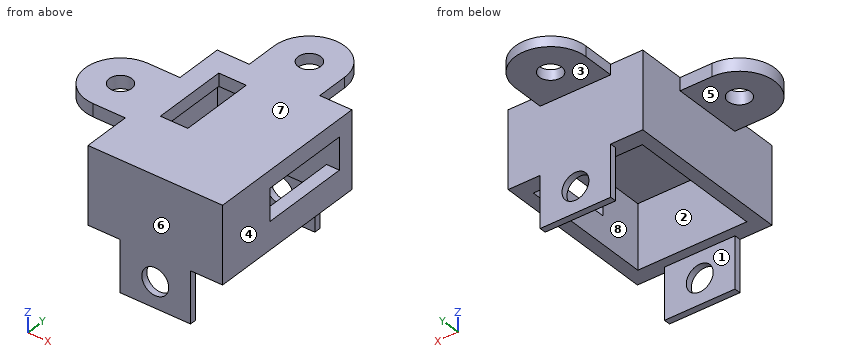
from build123d import *

# Parameters (mm, degrees)
SKETCH1_W           = 21
SKETCH1_H           = 26
SKETCH1_W_2         = 17
SKETCH1_H_2         = 21
BOSS_EXTRUDE1_DEPTH = 10
SKETCH2_W           = 21
SKETCH2_H           = 26
BOSS_EXTRUDE2_DEPTH = 2
SKETCH4_W           = 5
SKETCH4_H           = 14
CUT_EXTRUDE2_DEPTH  = 2
SKETCH6_R           = 1.76
BOSS_EXTRUDE3_DEPTH = 1.6
SKETCH9_R           = 1.76
BOSS_EXTRUDE5_DEPTH = 2
SKETCH14_W          = 11
SKETCH14_H          = 1
BOSS_EXTRUDE8_DEPTH = 8
SKETCH16_R          = 2.1
CUT_EXTRUDE3_DEPTH  = 39
CUT_EXTRUDE4_DEPTH  = 10
SKETCH18_R          = 1.75
BOSS_EXTRUDE9_DEPTH = 2
SKETCH19_W          = 4.280254221
SKETCH19_H          = 11.747931796
CUT_EXTRUDE5_DEPTH  = 10


with BuildPart() as part:
    # Sketch1 → Boss-Extrude1 (new body)
    with BuildSketch(Plane.XY):
        Rectangle(SKETCH1_W, SKETCH1_H)
        Rectangle(SKETCH1_W_2, SKETCH1_H_2, mode=Mode.SUBTRACT)
    extrude(amount=BOSS_EXTRUDE1_DEPTH)

    # Sketch2 → Boss-Extrude2 (add)
    with BuildSketch(Plane.XY.offset(10)):
        Rectangle(SKETCH2_W, SKETCH2_H)
    extrude(amount=BOSS_EXTRUDE2_DEPTH)

    # Sketch4 → Cut-Extrude2 (cut)
    with BuildSketch(Plane(origin=(10.5, 0, 0), x_dir=(0, 0, -1), z_dir=(1, 0, 0))):
        with Locations((-6.8, 3.5)):
            Rectangle(SKETCH4_W, SKETCH4_H)
    extrude(amount=-CUT_EXTRUDE2_DEPTH, mode=Mode.SUBTRACT)

    # Sketch6 → Boss-Extrude3 (add)
    with BuildSketch(Plane.XY.offset(12)):
        with BuildLine():
            Line((0, 13), (5.5, 13))
            Line((5.5, 13), (5.5, 18))
            ThreePointArc((5.5, 18), (0, 23.5), (-5.5, 18))
            Line((-5.5, 18), (-5.5, 13))
            Line((-5.5, 13), (0, 13))
        make_face()
        with Locations((0, 18)):
            Circle(SKETCH6_R, mode=Mode.SUBTRACT)
    extrude(amount=-BOSS_EXTRUDE3_DEPTH)

    # Sketch9 → Boss-Extrude5 (add)
    with BuildSketch(Plane.XY.offset(12)):
        with BuildLine():
            Line((0, -13), (-5.5, -13))
            Line((-5.5, -13), (-5.5, -18))
            ThreePointArc((-5.5, -18), (0, -23.5), (5.5, -18))
            Line((5.5, -18), (5.5, -13))
            Line((5.5, -13), (0, -13))
        make_face()
        with Locations((0, -18)):
            Circle(SKETCH9_R, mode=Mode.SUBTRACT)
    extrude(amount=-BOSS_EXTRUDE5_DEPTH)

    # Sketch14 → Boss-Extrude8 (add)
    with BuildSketch(Plane(origin=(0, 0, 0), x_dir=(-1, 0, 0), z_dir=(0, 0, -1))):
        with Locations((0, -12.5)):
            Rectangle(SKETCH14_W, SKETCH14_H)
        with Locations((0, 12.5)):
            Rectangle(SKETCH14_W, SKETCH14_H)
    extrude(amount=BOSS_EXTRUDE8_DEPTH)

    # Sketch16 → Cut-Extrude3 (cut)
    with BuildSketch(Plane(origin=(0, 13, 0), x_dir=(1, 0, 0), z_dir=(0, 1, 0))):
        with Locations((0, 4)):
            Circle(SKETCH16_R)
    extrude(amount=-CUT_EXTRUDE3_DEPTH, mode=Mode.SUBTRACT)

    # Sketch17 → Cut-Extrude4 (cut)
    with BuildSketch(Plane(origin=(0, 0, 10), x_dir=(-1, 0, 0), z_dir=(0, 0, -1))):
        with BuildLine():
            Line((-5.5, -18), (-5.5, -13))
            Line((-5.5, -13), (5.5, -13))
            Line((5.5, -13), (5.5, -18))
            ThreePointArc((5.5, -18), (0, -23.5), (-5.5, -18))
        make_face()
    extrude(amount=-CUT_EXTRUDE4_DEPTH, mode=Mode.SUBTRACT)

    # Sketch18 → Boss-Extrude9 (add)
    with BuildSketch(Plane.XY.offset(12)):
        with BuildLine():
            Line((-10.5, 0), (-10.5, 5.5))
            Line((-10.5, 5.5), (-15.5, 5.5))
            ThreePointArc((-15.5, 5.5), (-21, 0), (-15.5, -5.5))
            Line((-15.5, -5.5), (-10.5, -5.5))
            Line((-10.5, -5.5), (-10.5, 0))
        make_face()
        with Locations((-15.5, 0)):
            Circle(SKETCH18_R, mode=Mode.SUBTRACT)
    extrude(amount=-BOSS_EXTRUDE9_DEPTH)

    # Sketch19 → Cut-Extrude5 (cut)
    with BuildSketch(Plane(origin=(0, 0, 10), x_dir=(-1, 0, 0), z_dir=(0, 0, -1))):
        with Locations((5.165781479, 3.32004636)):
            Rectangle(SKETCH19_W, SKETCH19_H)
    extrude(amount=-CUT_EXTRUDE5_DEPTH, mode=Mode.SUBTRACT)


solid = part.part
Read the model definition and answer for the solid it produces. Units are mm, in the model's axes. Face numbers are marked on the shaded views. A direction names the side the tool comes from. Round coordinates to 2 decimals unless told otherwise and drop trailing zeros. Loops run counter-clockwise (first coordinate to the right, second up) from the corner with the lowest first, then second, coordinate; pieces in that order, holes last. Notation, with made-up numbers: (-0.5, 46) - (5.5, 46) arc R14 ccw to (5.5, 64) - close; hole circle Ø10 at (39, -5). An arc over 180 degrees is marked (long way). One line per question, with ' | ' between items. Start each with the question number.
Q1. For the marked faces 1, 2, 3, 4 and 5, determine the directions among +Z, -Z, +X, -X, +Y, -Y from which every point of the face is accessible in a straight line to the end or side of a thin tool.
Q2. Section D-D on x = 8 is taken. Give the vertices of the cut face in (y, z), plus the area to 3 significant figures.
Q3. For a pull along Y with two mould halves and no side action, classify the marked faces 6, 7 and 8 as +Y half, -Y half, draft (parallel to the pull), parting line (faces both ways), or undercut.
Q4. Section C-C on y = 4 is taken. Give the vertices of the cut face in (x, z).
Q5. Find the intervals of material crossed by L1, parallel to Y at x = -1, z = 9.5; L2, parallel to Z at x = 0, y = -12.35; L3, parallel to Y at x = -15.5, z = 10.95, in increasing order.
Q6. Section B-B on z = -3.25 is taken. Give the vertices of the cut face in (x, y), plus the area to 3 significant figures.
Q7. Section A-A on y = 0 is taken. Give the vertices of the cut face in (x, z), plus the area to 3 significant figures.
Q8. Flat-ended cylindrical pins translate along their axes: pin 1 (9 mm diameter, centred on x = 1.5, z = -5.5, fed in from +Y); pin 2 (1.5 mm diameter, centred on x = -10.5, y = -3.5, fed in from -Z); pin 3 (1 mm diameter, centred on x = -13, z = 11, fed in from +Y). Find the tip coordinate at first contact, or state that the pin passes through.
Established:
1) face 1: -Z, +X, -X | face 2: -Z | face 3: -Z, +X, -X, +Y | face 4: +Z, -Z, +X, +Y, -Y | face 5: -Z, -X, +Y, -Y
2) outline: (-13, 0) - (-10.5, 0) - (-10.5, 10) - (10.5, 10) - (10.5, 0) - (13, 0) - (13, 12) - (-13, 12) - close | area: 102 mm²
3) face 6: -Y half | face 7: draft | face 8: undercut
4) outline: (-19.27, 10) - (-10.5, 10) - (-10.5, 0) - (-8.5, 0) - (-8.5, 10) - (-7.31, 10) - (-7.31, 12) - (-19.27, 12) - close; (-3.03, 10) - (8.5, 10) - (8.5, 9.3) - (10.5, 9.3) - (10.5, 12) - (-3.03, 12) - close; (8.5, 0) - (10.5, 0) - (10.5, 4.3) - (8.5, 4.3) - close
5) L1: -13 to -10.5, 10.5 to 13 | L2: -8 to -6.1, -1.9 to 12 | L3: -5.5 to -1.75, 1.75 to 5.5
6) outline: (-5.5, -13) - (-1.96, -13) - (-1.96, -12) - (-5.5, -12) - close; (-5.5, 12) - (-1.96, 12) - (-1.96, 13) - (-5.5, 13) - close; (1.96, -13) - (5.5, -13) - (5.5, -12) - (1.96, -12) - close; (1.96, 12) - (5.5, 12) - (5.5, 13) - (1.96, 13) - close | area: 14.2 mm²
7) outline: (-21, 10) - (-17.25, 10) - (-17.25, 12) - (-21, 12) - close; (-13.75, 10) - (-10.5, 10) - (-10.5, 0) - (-8.5, 0) - (-8.5, 10) - (-7.31, 10) - (-7.31, 12) - (-13.75, 12) - close; (-3.03, 10) - (8.5, 10) - (8.5, 9.3) - (10.5, 9.3) - (10.5, 12) - (-3.03, 12) - close; (8.5, 0) - (10.5, 0) - (10.5, 4.3) - (8.5, 4.3) - close | area: 77.4 mm²
8) pin 1: y = 13 | pin 2: z = 0 | pin 3: y = 5.5
